The model under review builds one solid part; all positions refer to its coordinate system, in mm. A direction names the side the tool comes from. Give positions to 0.01 mm unless a question says otherwise; leave off trailing zeros. Loops run counter-clockwise (first coordinate to the right, second up) from the corner with the lowest first, then second, coordinate; pieces in that order, holes last. Notation, with made-up numbers: (41, 39.25) - (80, 39.25) arc R14 cw to (80, 52.25) - close; hole circle Ø4 at (-1.75, 44). An arc over 180 degrees is marked (long way). Answer as a JSON object with one key per item and string values.
from build123d import *

# Parameters (mm, degrees)
SKETCH1_W           = 42
SKETCH1_H           = 35
BOSS_EXTRUDE1_DEPTH = 4
FILLET1_R           = 1
FILLET2_R           = 1
SKETCH2_R           = 0.5
SKETCH5_R           = 0.5
SKETCH10_R          = 0.3
SKETCH13_R          = 0.3
BOSS_EXTRUDE2_DEPTH = 4


with BuildPart() as part:
    # Sketch1 → Boss-Extrude1 (new body)
    with BuildSketch(Plane(origin=(0, 0, 0), x_dir=(1, 0, 0), z_dir=(0, 1, 0))):
        with Locations((21, 17.5)):
            Rectangle(SKETCH1_W, SKETCH1_H)
    extrude(amount=BOSS_EXTRUDE1_DEPTH)

    # Fillet1
    fillet1_edges = [part.edges().sort_by_distance(p)[0] for p in [
        (0, 2, 0),
        (42, 2, 0),
        (42, 2, -35),
        (0, 2, -35),
    ]]
    fillet(fillet1_edges, radius=FILLET1_R)

    # Fillet2
    fillet2_edges = [part.edges().sort_by_distance(p)[0] for p in [
        (42, 0, -17.5),
        (42, 4, -17.5),
        (0, 0, -17.5),
        (21, 0, -35),
        (21, 0, 0),
        (0.292893219, 0, -0.292893219),
        (0.292893219, 0, -34.707106781),
        (41.707106781, 0, -34.707106781),
        (41.707106781, 0, -0.292893219),
        (21, 4, 0),
        (0, 4, -17.5),
        (21, 4, -35),
        (0.292893219, 4, -0.292893219),
        (0.292893219, 4, -34.707106781),
        (41.707106781, 4, -34.707106781),
        (41.707106781, 4, -0.292893219),
    ]]
    fillet(fillet2_edges, radius=FILLET2_R)

    # Sweep2: sweep along a path in Sketch4
    with BuildLine(Plane(origin=(0, 0, 0), x_dir=(1, 0, 0), z_dir=(0, 1, 0))) as sweep2_path:
        Line((42, 32.598834146), (43.472011027, 32.598834146))
        ThreePointArc((43.472011027, 32.598834146), (46.584840442, 31.309457985), (47.874216603, 28.19662857))
        Line((47.874216603, 28.19662857), (47.874216603, 16.805737351))
    # Sketch2 → Sweep2 (sweep)
    with BuildSketch(Plane(origin=(42, 0, 0), x_dir=(0, 0, -1), z_dir=(1, 0, 0))):
        with Locations((32.598834146, 2)):
            Circle(SKETCH2_R)
    sweep(path=sweep2_path.line)

    # Sweep3: sweep along a path in Sketch6
    with BuildLine(Plane(origin=(0, 0, 0), x_dir=(1, 0, 0), z_dir=(0, 1, 0))) as sweep3_path:
        Line((42, 30.237830041), (42.053967758, 30.237830041))
        ThreePointArc((42.053967758, 30.237830041), (43.992158066, 29.435005329), (44.794982779, 27.49681502))
        Line((44.794982779, 27.49681502), (44.794982779, 20.415467716))
    # Sketch5 → Sweep3 (sweep)
    with BuildSketch(Plane(origin=(42, 0, 0), x_dir=(0, 0, -1), z_dir=(1, 0, 0))):
        with Locations((30.237830041, 2)):
            Circle(SKETCH5_R)
    sweep(path=sweep3_path.line)

    # Sweep5: sweep along a path in Sketch12
    with BuildLine(Plane(origin=(44.828772476, 0, 0), x_dir=(0, 0, -1), z_dir=(1, 0, 0))) as sweep5_path:
        Line((20.415467716, 2), (20.413075866, 2))
        ThreePointArc((20.413075866, 2), (20.200943832, 1.912132034), (20.113075866, 1.7))
        Line((20.113075866, 1.7), (20.113075866, -1.34465824))
    # Sketch10 → Sweep5 (sweep)
    with BuildSketch(Plane.XY.offset(-20.415467716)):
        with Locations((44.794982779, 2)):
            Circle(SKETCH10_R)
    sweep(path=sweep5_path.line)

    # Sketch13 → Boss-Extrude2 (add)
    with BuildSketch(Plane.XY.offset(-16.805737351)):
        with Locations((47.874216603, 2)):
            Circle(SKETCH13_R)
    extrude(amount=BOSS_EXTRUDE2_DEPTH)


solid = part.part
Q1. The part is to be moulded in two halves that separate along X. For faces 1 (the face through (0.301, 0.285, -17.269)), 2 (the face through (41.699, 2.014, -0.285)), 3 (the face through (44.295, 2.022, -23.907)), say which applies: +X half, -X half, draft (parallel to the pull), parting line (faces both ways), or undercut.
Results:
{"face 1": "-X half", "face 2": "+X half", "face 3": "undercut"}
Q2. To check wall thickness, follow probe 1 along Y at (x, z) = (27, -10.5); probe 2 along X at (y, z) = (2.3, -6.5); probe 3 along Z at (x, y) = (27.5, 3.2). State the ranges of each line that lie inside material, in increasing order. Write a range as [from, to].
Results:
{"probe 1": "y = [0, 4]", "probe 2": "x = [0, 42]", "probe 3": "z = [-34.98, -0.02]"}
Q3. Consider section A-A, the plane z = -18. State the section outline as (x, y) points, plus the area to 3 significant figures.
Results:
{"outline": "(0, 1) arc R1 ccw to (1, 0) - (41, 0) arc R1 ccw to (42, 1) - (42, 3) arc R1 ccw to (41, 4) - (1, 4) arc R1 ccw to (0, 3) - close; circle Ø1 at (47.87, 2)", "area": "168 mm^2"}
Q4. For faces 4 (the face through (47.375, 2.022, -22.421)), 5 (the face through (21.28, 3.715, -0.301)), 6 (the face through (42.746, 2.15, -33.076)), list the 3-axis set-ups (+Z, -Z, +X, -X, +Y, -Y) from which the entire face can be reached by the end or side of a thin tool; tool diameter is ignored.
Results:
{"face 4": "+Z", "face 5": "+Z, +X, -X, +Y", "face 6": "none"}
Q5. Consider section B-B, the plane z = -6.5. State the section outline as (x, y) points.
Results:
{"outline": "(0, 1) arc R1 ccw to (1, 0) - (41, 0) arc R1 ccw to (42, 1) - (42, 3) arc R1 ccw to (41, 4) - (1, 4) arc R1 ccw to (0, 3) - close"}
Q6. Clearance check with a flat-ended pin moving along its axis: pin 1 Ø0.8 at (x, y) = (48, 2) entering from +Z. State where the tip first meets the part, or that it passes through.
Results:
{"pin 1": "stops at z = -12.81"}
Q7. Consider section C-C, the plane x = 33.5. State the section outline as (y, z) points, plus the area to 3 significant figures.
Results:
{"outline": "(0, -34) arc R1 ccw to (1, -35) - (3, -35) arc R1 ccw to (4, -34) - (4, -1) arc R1 ccw to (3, 0) - (1, 0) arc R1 ccw to (0, -1) - close", "area": "139 mm^2"}
